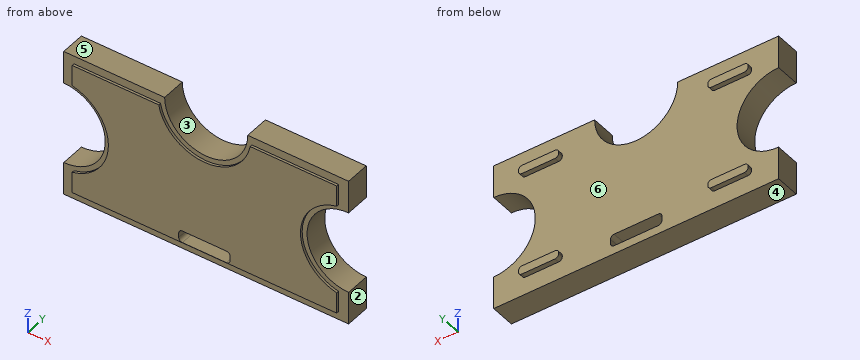
```python
from build123d import *

# Parameters (mm, degrees)
F1_DEPTH = 20
F3_DEPTH = 2
F5_DEPTH = 4
F6_DEPTH = 4


with BuildPart() as f1:
    # F0 (on Front) → F1 (new body)
    with BuildSketch(Plane.XZ):
        with BuildLine():
            Line((116.590939, 34), (116.590939, 61.067935))
            Line((116.590939, 61.067935), (34, 61.067935))
            ThreePointArc((34, 61.067935), (0, 27.067935), (-34, 61.067935))
            Line((-34, 61.067935), (-116.590939, 61.067935))
            Line((-116.590939, 61.067935), (-116.590939, 34))
            ThreePointArc((-116.590939, 34), (-82.590939, 0), (-116.590939, -34))
            Line((-116.590939, -34), (-116.590939, -61.067935))
            Line((-116.590939, -61.067935), (34, -61.067935))
            Line((34, -61.067935), (116.590939, -61.067935))
            Line((116.590939, -61.067935), (116.590939, -34))
            ThreePointArc((116.590939, -34), (82.590939, 0), (116.590939, 34))
        make_face()
        with BuildLine():
            Line((-18.030702, -44.351537), (18.030702, -44.351537))
            ThreePointArc((18.030702, -44.351537), (20.152022, -45.230216), (21.030702, -47.351537))
            Line((21.030702, -47.351537), (21.030702, -51.243211))
            ThreePointArc((21.030702, -51.243211), (20.152022, -53.364531), (18.030702, -54.243211))
            Line((18.030702, -54.243211), (-18.030702, -54.243211))
            ThreePointArc((-18.030702, -54.243211), (-20.152022, -53.364531), (-21.030702, -51.243211))
            Line((-21.030702, -51.243211), (-21.030702, -47.351537))
            ThreePointArc((-21.030702, -47.351537), (-20.152022, -45.230216), (-18.030702, -44.351537))
        make_face(mode=Mode.SUBTRACT)
    extrude(amount=-F1_DEPTH)

    # F2 (on face) → F3 (join)
    with BuildSketch(Plane.XZ):
        with BuildLine():
            Line((108.294822, 37.083345), (108.294822, 54.408085))
            Line((108.294822, 54.408085), (37.411848, 54.408085))
            ThreePointArc((37.411848, 54.408085), (0, 23.067935), (-37.411848, 54.408085))
            Line((-37.411848, 54.408085), (-108.294822, 54.408085))
            Line((-108.294822, 54.408085), (-108.294822, 37.083345))
            ThreePointArc((-108.294822, 37.083345), (-78.590939, 0), (-108.294822, -37.083345))
            Line((-108.294822, -37.083345), (-108.294822, -54.408085))
            Line((-108.294822, -54.408085), (108.294822, -54.408085))
            Line((108.294822, -54.408085), (108.294822, -37.083345))
            ThreePointArc((108.294822, -37.083345), (78.590939, 0), (108.294822, 37.083345))
        make_face()
        with BuildLine():
            Line((-21.030702, -51.243211), (-21.030702, -47.351537))
            ThreePointArc((-21.030702, -47.351537), (-20.152022, -45.230216), (-18.030702, -44.351537))
            Line((-18.030702, -44.351537), (18.030702, -44.351537))
            ThreePointArc((18.030702, -44.351537), (20.152022, -45.230216), (21.030702, -47.351537))
            Line((21.030702, -47.351537), (21.030702, -51.243211))
            ThreePointArc((21.030702, -51.243211), (20.152022, -53.364531), (18.030702, -54.243211))
            Line((18.030702, -54.243211), (-18.030702, -54.243211))
            ThreePointArc((-18.030702, -54.243211), (-20.152022, -53.364531), (-21.030702, -51.243211))
        make_face(mode=Mode.SUBTRACT)
    extrude(amount=F3_DEPTH)

    # F4 (on face) → F5 (join)
    with BuildSketch(Plane(origin=(0, 20, 0), x_dir=(-1, 0, 0), z_dir=(0, 1, 0))):
        with BuildLine():
            ThreePointArc((-60.5, 43.5), (-61.37868, 45.62132), (-63.5, 46.5))
            Line((-63.5, 46.5), (-90.5, 46.5))
            ThreePointArc((-90.5, 46.5), (-92.62132, 45.62132), (-93.5, 43.5))
            Line((-93.5, 43.5), (-93.5, 42.5))
            ThreePointArc((-93.5, 42.5), (-92.62132, 40.37868), (-90.5, 39.5))
            Line((-90.5, 39.5), (-63.5, 39.5))
            ThreePointArc((-63.5, 39.5), (-61.37868, 40.37868), (-60.5, 42.5))
            Line((-60.5, 42.5), (-60.5, 43.5))
        make_face()
    extrude(amount=F5_DEPTH)

    # F4 (on face) → F6 (join)
    with BuildSketch(Plane(origin=(0, 20, 0), x_dir=(-1, 0, 0), z_dir=(0, 1, 0))):
        with BuildLine():
            ThreePointArc((-60.5, 43.5), (-61.37868, 45.62132), (-63.5, 46.5))
            Line((-63.5, 46.5), (-90.5, 46.5))
            ThreePointArc((-90.5, 46.5), (-92.62132, 45.62132), (-93.5, 43.5))
            Line((-93.5, 43.5), (-93.5, 42.5))
            ThreePointArc((-93.5, 42.5), (-92.62132, 40.37868), (-90.5, 39.5))
            Line((-90.5, 39.5), (-63.5, 39.5))
            ThreePointArc((-63.5, 39.5), (-61.37868, 40.37868), (-60.5, 42.5))
            Line((-60.5, 42.5), (-60.5, 43.5))
        make_face()
        with BuildLine():
            ThreePointArc((-60.5, -42.5), (-61.37868, -40.37868), (-63.5, -39.5))
            Line((-63.5, -39.5), (-90.5, -39.5))
            ThreePointArc((-90.5, -39.5), (-92.62132, -40.37868), (-93.5, -42.5))
            Line((-93.5, -42.5), (-93.5, -43.5))
            ThreePointArc((-93.5, -43.5), (-92.62132, -45.62132), (-90.5, -46.5))
            Line((-90.5, -46.5), (-63.5, -46.5))
            ThreePointArc((-63.5, -46.5), (-61.37868, -45.62132), (-60.5, -43.5))
            Line((-60.5, -43.5), (-60.5, -42.5))
        make_face()
        with BuildLine():
            Line((91.5, 46.5), (64.5, 46.5))
            ThreePointArc((64.5, 46.5), (62.37868, 45.62132), (61.5, 43.5))
            Line((61.5, 43.5), (61.5, 42.5))
            ThreePointArc((61.5, 42.5), (62.37868, 40.37868), (64.5, 39.5))
            Line((64.5, 39.5), (91.5, 39.5))
            ThreePointArc((91.5, 39.5), (93.62132, 40.37868), (94.5, 42.5))
            Line((94.5, 42.5), (94.5, 43.5))
            ThreePointArc((94.5, 43.5), (93.62132, 45.62132), (91.5, 46.5))
        make_face()
        with BuildLine():
            Line((91.5, -39.5), (64.5, -39.5))
            ThreePointArc((64.5, -39.5), (62.37868, -40.37868), (61.5, -42.5))
            Line((61.5, -42.5), (61.5, -43.5))
            ThreePointArc((61.5, -43.5), (62.37868, -45.62132), (64.5, -46.5))
            Line((64.5, -46.5), (91.5, -46.5))
            ThreePointArc((91.5, -46.5), (93.62132, -45.62132), (94.5, -43.5))
            Line((94.5, -43.5), (94.5, -42.5))
            ThreePointArc((94.5, -42.5), (93.62132, -40.37868), (91.5, -39.5))
        make_face()
    extrude(amount=F6_DEPTH)


solid = f1.part
```
Can you work these out from the model? Positions are in its coordinate system, mm. Face numbers are marked on the shaded views. A direction names the side the tool comes from. Give positions to 0.01 mm unless a question says otherwise; leave off trailing zeros. Order: outer loops, then holes, each group sorted by start corner. A loop starts at its lowest first (then second) coordinate and runs counter-clockwise, first axis right, second up. Notation, with made-up numbers: (39.25, 59) - (71.25, 59) arc R27 cw to (71.25, 94) - close; hole circle Ø5 at (23, 78.25). An arc over 180 degrees is marked (long way). Use a Markdown table: item, result. Add a question column.
Q1. If we mould it in two halves opening along Z, with no side actions, what happens to the marked faces 1, 2, 3 and 4? For each: released by +Z, released by -Z, zero draft, split by the parting line, or undercut.
Q2. I'm going to push flat-ended pins straight in: pin 1 (12 mm diameter, centred on y = 1.5, z = 11.5, fed in from +X); pin 2 (10 mm diameter, centred on x = -23, y = 9.5, fed in from +Z); pin 3 (3 mm diameter, centred on y = 20, z = 13.5, fed in from -X). Where does each tip first touch, or does it pass through?
Q3. Please list where these lines run through material, in increasing order: line 1 along X through (y, z) = (-0.25, 53); line 2 along Y through (x, z) = (40, 39.5); line 3 along X through (y, z) = (-0.5, 47).
Q4. If we section it at C-C on z = 0: Write out the boundary of the cut face in (x, y).
Q5. On a 3-axis mill with a long thin cutter (end or side, diameter ignored), from which of +Z, -Z, +X, -X, +Y, -Y can I reach the whole of each face in a straight line? I mean the marked faces 5 and 6. Say none if no direction works.
Q6. If we section it at B-B on y = 13.75: Write out the boundary of the cut face in (x, z).
Q7. If we section it at D-D on x = 43: Write out the boundary of the cut face in (y, z), plus the area to 3 significant figures.
Q8. If we section it at A-A on x = 0: Write out the boundary of the cut face in (y, z), plus the area to 3 significant figures.
Answers follow:
| question | item | result |
|---|---|---|
| 1 | face 1 | undercut |
| 1 | face 2 | zero draft |
| 1 | face 3 | released by +Z |
| 1 | face 4 | released by -Z |
| 2 | pin 1 | stops at x = 87.44 |
| 2 | pin 2 | stops at z = 41.78 |
| 2 | pin 3 | stops at x = -86.08 |
| 3 | line 1 | x = -108.29 to -37.13, 37.13 to 108.29 |
| 3 | line 2 | y = -2 to 20 |
| 3 | line 3 | x = -108.29 to -35.3, 35.3 to 108.29 |
| 4 | outline | (-82.59, 0) - (-78.59, 0) - (-78.59, -2) - (78.59, -2) - (78.59, 0) - (82.59, 0) - (82.59, 20) - (-82.59, 20) - close |
| 5 | face 5 | +Z, +X, -X, +Y, -Y |
| 5 | face 6 | +Y |
| 6 | outline | (-116.59, -61.07) - (116.59, -61.07) - (116.59, -34) arc R34 cw to (116.59, 34) - (116.59, 61.07) - (34, 61.07) arc R34 cw to (-34, 61.07) - (-116.59, 61.07) - (-116.59, 34) arc R34 cw to (-116.59, -34) - close; hole (-21.03, -51.24) arc R3 ccw to (-18.03, -54.24) - (18.03, -54.24) arc R3 ccw to (21.03, -51.24) - (21.03, -47.35) arc R3 ccw to (18.03, -44.35) - (-18.03, -44.35) arc R3 ccw to (-21.03, -47.35) - close |
| 7 | outline | (-2, -54.41) - (0, -54.41) - (0, -61.07) - (20, -61.07) - (20, 61.07) - (0, 61.07) - (0, 54.41) - (-2, 54.41) - close |
| 7 | area | 2,660 mm^2 |
| 8 | outline | (-2, -54.41) - (0, -54.41) - (0, -61.07) - (20, -61.07) - (20, -54.24) - (-2, -54.24) - close; (-2, -44.35) - (20, -44.35) - (20, 27.07) - (0, 27.07) - (0, 23.07) - (-2, 23.07) - close |
| 8 | area | 1,700 mm^2 |
